from build123d import *

# Parameters (mm, degrees)
F1_DEPTH = 5
F2_R     = 0.65
F3_DEPTH = 7
F4_SIZE  = 1


with BuildPart() as f1:
    # F0 (on Front) → F1 (new body)
    with BuildSketch(Plane.XZ):
        Polygon((-36.916861, 60.554342), (-41.916861, 60.554342), (-41.916861, -4.445658), (-36.916861, -4.445658), (-29.416861, -4.445658), (-29.416861, 15.554342), (-36.916861, 15.554342), align=None)
    extrude(amount=F1_DEPTH)

    # F2 (on face) → F3 (cut)
    with BuildSketch(Plane.XY.offset(60.554342)):
        with Locations((-39.416861, -2.5)):
            Circle(F2_R)
    extrude(amount=-F3_DEPTH, mode=Mode.SUBTRACT)

    # F4
    f4_edges = [f1.edges().sort_by_distance(p)[0] for p in [
        (-36.916861, -2.5, 60.554342),
        (-39.416861, -5, 60.554342),
        (-39.416861, 0, 60.554342),
        (-41.916861, -2.5, 60.554342),
    ]]
    chamfer(f4_edges, length=F4_SIZE)


solid = f1.part
Check sheet for the modelled part. Datum: model origin and axes. Units: mm. A direction names the side the tool comes from. Give positions to 0.01 mm unless a question says otherwise; leave off trailing zeros. Order: outer loops, then holes, each group sorted by start corner. A loop starts at its lowest first (then second) coordinate and runs counter-clockwise, first axis right, second up. Notation, with made-up numbers: M 59.25,-24 L 84.25,-24 A25 ccw 84.25,-12 Z; hole C -8.5,-32 d2. An arc over 180 degrees is marked long. Answer as CSV lines item,"result". Start each with the question number.
Item 1: Cross-section at A-A on y = -2.5. Enter the section's corners in (x, z), plus the area to 3 significant figures.
Item 2: Thickness scan on line 1 (X direction, y = -0.95, z = 47); line 2 (Z direction, x = -33.25, y = -3.3); line 3 (Z direction, x = -37, y = -1.7). Record the ranges inside material, lowest first. Write a range as [from, to].
Item 3: Cross-section at C-C on x = -34.5. Enter the section's corners in (y, z).
Item 4: Tool access check on faces 4 (the face through (-39.382, -4.507, 60.047)), 5 (the face through (-33, -2, 15.554)), 6 (the face through (-39.4, -2.5, 53.554)). Record the directions out of +Z, -Z, +X, -X, +Y, -Y that give a thin tool (end or side, any length) a straight path to the whole face; none if there is none.
Item 5: Mould release check, pull along X, two halves, no side actions. Record for faces 1 (the face through (-29.417, -2, 5)), 2 (the face through (-40.066, -2.471, 57.103)), 3 (the face through (-38.7, -2.1, 60.554)): +X half, -X half, draft (parallel to the pull), parting line (faces both ways), or undercut.
Item 6: Cross-section at B-B on z = 52. Enter the section's corners in (x, y), plus the area to 3 significant figures.
Established:
1,outline,"M -41.92,-4.45 L -29.42,-4.45 L -29.42,15.55 L -36.92,15.55 L -36.92,59.55 L -37.92,60.55 L -38.77,60.55 L -38.77,53.55 L -40.07,53.55 L -40.07,60.55 L -40.92,60.55 L -41.92,59.55 Z"
1,area,"465 mm^2"
2,line 1,"x = [-41.92, -36.92]"
2,line 2,"z = [-4.45, 15.55]"
2,line 3,"z = [-4.45, 59.64]"
3,outline,"M -5,-4.45 L 0,-4.45 L 0,15.55 L -5,15.55 Z"
4,face 4,"+Z, +X, -X, -Y"
4,face 5,"+Z, +X, +Y, -Y"
4,face 6,"+Z"
5,face 1,"+X half"
5,face 2,"undercut"
5,face 3,"draft"
6,outline,"M -41.92,-5 L -36.92,-5 L -36.92,0 L -41.92,0 Z"
6,area,"25.0 mm^2"
